from build123d import *

# Parameters (mm, degrees)
SKETCH1_R           = 2.5
BOSS_EXTRUDE1_DEPTH = 25
CUT_EXTRUDE2_DEPTH  = 22


with BuildPart() as part:
    # Sketch1 → Boss-Extrude1 (new body)
    with BuildSketch(Plane(origin=(0, 0, 0), x_dir=(1, 0, 0), z_dir=(0, 1, 0))):
        Polygon((-29.5, 28), (35.5, 28), (35.5, -28), (-29.5, -28), (-29.5, -53), (-65.5, -53), (-65.5, 53), (-29.5, 53), align=None)
        with Locations((-25, 17.5)):
            Circle(SKETCH1_R, mode=Mode.SUBTRACT)
        with Locations((25, 17.5)):
            Circle(SKETCH1_R, mode=Mode.SUBTRACT)
        with Locations((25, -17.5)):
            Circle(SKETCH1_R, mode=Mode.SUBTRACT)
        with Locations((-25, -17.5)):
            Circle(SKETCH1_R, mode=Mode.SUBTRACT)
    extrude(amount=BOSS_EXTRUDE1_DEPTH)

    # Sketch6 → Cut-Extrude2 (cut)
    with BuildSketch(Plane(origin=(0, 25, 0), x_dir=(1, 0, 0), z_dir=(0, 1, 0))):
        Polygon((-32.5, 25), (-32.5, 50), (-62.5, 50), (-62.5, -50), (-32.5, -50), (-32.5, -25), (32.5, -25), (32.5, 25), align=None)
    extrude(amount=-CUT_EXTRUDE2_DEPTH, mode=Mode.SUBTRACT)


solid = part.part
Can you work these out from the model? Positions are in its coordinate system, mm. A direction names the side the tool comes from. Coordinates: 2 decimals unless noted, no trailing zeros. Write each loop counter-clockwise with the first axis right and the second up, starting at its lowest first coordinate (ties: lowest second). Pieces come first, ordered by that corner, then holes. Notation, with made-up numbers: (16.5, -2.5) -> (61.5, -2.5) arc R33 cw to (61.5, 31.5) -> close; hole circle Ø8 at (60.25, 19). An arc over 180 degrees is marked (long way). Write item = value, one per line.
(1) Imagine slicing it at B-B (y = 6.5). Please give me the cut outline in (x, z).
Verdict:
outline = (-65.5, -53) -> (-29.5, -53) -> (-29.5, -28) -> (35.5, -28) -> (35.5, 28) -> (-29.5, 28) -> (-29.5, 53) -> (-65.5, 53) -> close; hole (-62.5, -50) -> (-32.5, -50) -> (-32.5, -25) -> (32.5, -25) -> (32.5, 25) -> (-32.5, 25) -> (-32.5, 50) -> (-62.5, 50) -> close
(2) For pin 1 (6 mm diameter, centred on x = 25, z = -17.5, fed in from +Y); pin 2 (6.5 mm diameter, centred on x = 5, y = 18, fed in from -Z); pin 3 (6 mm diameter, centred on y = 2.5, z = 39.5, fed in from +X), each with a flat end and sliding along its axis, tell me the tip position at first contact or that it passes through.
Verdict:
pin_1 = 3
pin_2 = -28
pin_3 = -29.5
(3) Thinking about a two-plate mould opening in Z: for faces 5 (the face through (-65.5, 12, 1)), 6 (the face through (-47, 12, 53)), 7 (the face through (-32.5, 14, -37)), which applies, +Z half, -Z half, draft (parallel to the pull), parting line (faces both ways), or undercut?
Verdict:
face_5 = draft
face_6 = +Z half
face_7 = undercut
(4) Imagine slicing it at A-A (z = -17.5). Please give me the cut outline in (x, y).
Verdict:
outline = (-65.5, 0) -> (-27.5, 0) -> (-27.5, 3) -> (-62.5, 3) -> (-62.5, 25) -> (-65.5, 25) -> close; (-22.5, 0) -> (22.5, 0) -> (22.5, 3) -> (-22.5, 3) -> close; (27.5, 0) -> (35.5, 0) -> (35.5, 25) -> (32.5, 25) -> (32.5, 3) -> (27.5, 3) -> close
(5) Imagine slicing it at C-C (x = 25). Please give me the cut outline in (y, z).
Verdict:
outline = (0, -28) -> (25, -28) -> (25, -25) -> (3, -25) -> (3, -20) -> (0, -20) -> close; (0, -15) -> (3, -15) -> (3, 15) -> (0, 15) -> close; (0, 20) -> (3, 20) -> (3, 25) -> (25, 25) -> (25, 28) -> (0, 28) -> close
(6) If I drill on probe 1 along X at (y, z) = (1.75, 17.5); probe 2 along X at (y, z) = (23.75, 37); probe 3 along X at (y, z) = (4.75, -12), over which ranges is the centre line in solid material (lowest first)?
Verdict:
probe_1 = -65.5 to -27.5, -22.5 to 22.5, 27.5 to 35.5
probe_2 = -65.5 to -62.5, -32.5 to -29.5
probe_3 = -65.5 to -62.5, 32.5 to 35.5
(7) On a 3-axis mill with a long thin cutter (end or side, diameter ignored), from which of +Z, -Z, +X, -X, +Y, -Y can I reach the whole of each face in a straight line? I mean faces 1 (the face through (0, 14, 25)), 2 (the face through (-22, 25, 27)), 3 (the face through (3, 12, -28)), 4 (the face through (-29.5, 12, 40)). Say none if no direction works.
Verdict:
face_1 = +Y
face_2 = +Z, -Z, +X, -X, +Y
face_3 = -Z, +X, +Y, -Y
face_4 = +Z, +X, +Y, -Y
(8) Imagine slicing it at D-D (x = -55.5). Please give me the cut outline in (y, z), and give its area (3 significant figures).
Verdict:
outline = (0, -53) -> (25, -53) -> (25, -50) -> (3, -50) -> (3, 50) -> (25, 50) -> (25, 53) -> (0, 53) -> close
area = 450 mm^2
